Here's the drawing with two shaded views (mm, measured from the low corner). I have some questions. A direction names the side the tool comes from. Give positions to 0.01 mm unless a question says otherwise; leave off trailing zeros. Loops run counter-clockwise (first coordinate to the right, second up) from the corner with the lowest first, then second, coordinate; pieces in that order, holes last. Notation, with made-up numbers: M 18.5,34.25 L 59.5,34.25 A25 ccw 59.5,52.25 Z; hole C 36,66.5 d3. An arc over 180 degrees is marked long. Write item = value, one per line. Start each with the question number.
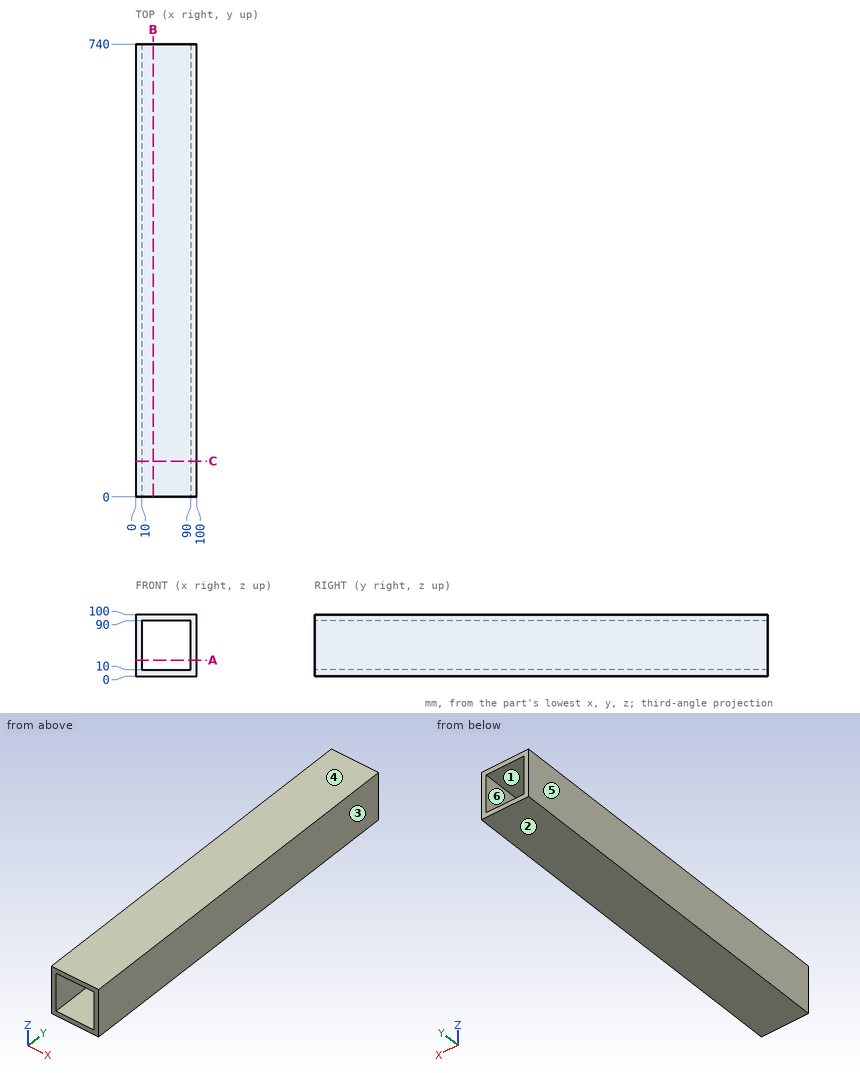
Q1. If I drill on line 1 along Z through (x, y) = (70, 585.5), over which ranges is the centre line in solid material (lowest first)?
Q2. On a 3-axis mill with a long thin cutter (end or side, diameter ignored), from which of +Z, -Z, +X, -X, +Y, -Y can I reach the whole of each face in a straight line? I mean the marked faces 5 and 6. Say none if no direction works.
Q3. If we section it at B-B, the plane x = 29: List the corners of the cut face in (y, z) for me, then the cut area to 3 significant figures.
Q4. If we section it at A-A, the plane z = 26: List the corners of the cut face in (x, y) for me.
Q5. We'd pull the mould along Z, two halves only. Please class the marked faces 1, 2, 3 and 4: pulls with the +Z half, pulls with the -Z half, needs draft (parallel to the pull), parting line crosses it, or undercut.
Q6. Will these pins go through, and if not, where does the flat tip stop? pin 1 (3 mm diameter, centred on x = 55.5, z = 87, fed in from -Y); pin 2 (5 mm diameter, centred on x = 37, y = 501.5, fed in from -Z).
Q7. If we section it at C-C, the plane y = 58.5: List the corners of the cut face in (x, z) for me, then the cut area to 3 significant figures.
Resolved:
q1.line_1 = 0 to 10, 90 to 100
q2.face_5 = +Z, -Z, -X, +Y, -Y
q2.face_6 = +Y, -Y
q3.outline = M 0,0 L 740,0 L 740,10 L 0,10 Z; M 0,90 L 740,90 L 740,100 L 0,100 Z
q3.area = 14,800 mm²
q4.outline = M 0,0 L 10,0 L 10,740 L 0,740 Z; M 90,0 L 100,0 L 100,740 L 90,740 Z
q5.face_1 = undercut
q5.face_2 = pulls with the -Z half
q5.face_3 = needs draft
q5.face_4 = pulls with the +Z half
q6.pin_1 = through
q6.pin_2 = 0
q7.outline = M 0,0 L 100,0 L 100,100 L 0,100 Z; hole M 10,10 L 90,10 L 90,90 L 10,90 Z
q7.area = 3,600 mm²
